from build123d import *

# Parameters (mm, degrees)
CROQUIS2_R            = 1.7
CORTAR_EXTRUIR1_DEPTH = 59
MATRIZC1_COUNT        = 3


with BuildPart() as part:
    # Croquis1 → Revolución1 (revolve)
    with BuildSketch(Plane.XY):
        Polygon((58.282962044, 6), (58.282962044, 0), (75, 0), (75, 27.5), (55, 27.5), (55, 13), (49, 13), (49, 12.5), align=None)
    revolve(axis=Axis((0, 0, 0), (0, 1, 0)))

    # Croquis2 → Cortar-Extruir1 (cut)
    with BuildSketch(Plane(origin=(0, 27.5, 0), x_dir=(1, 0, 0), z_dir=(0, 1, 0))):
        with Locations((-65, 0)):
            Circle(CROQUIS2_R)
    cortar_extruir1 = extrude(amount=-CORTAR_EXTRUIR1_DEPTH, mode=Mode.SUBTRACT)

    # MatrizC1: Cortar-Extruir1 ×3 about axis
    matrizc1_axis = Axis((0, 0, 0), (0, 1, 0))
    for i in range(1, MATRIZC1_COUNT):
        add(cortar_extruir1.rotate(matrizc1_axis, i * 360 / MATRIZC1_COUNT), mode=Mode.SUBTRACT)


solid = part.part
Design review of the part built by this model. Coordinates are the model's own, in mm. A direction names the side the tool comes from. Coordinates: 2 decimals unless noted, no trailing zeros. Loops run counter-clockwise (first coordinate to the right, second up) from the corner with the lowest first, then second, coordinate; pieces in that order, holes last.
Item 1: Clearance check with flat-ended pins moving along their axes: pin 1 (4 mm diameter, centred on x = -18.5, y = 16.5, fed in from +Z); pin 2 (10 mm diameter, centred on y = 20.5, z = 31.5, fed in from -X); pin 3 (5 mm diameter, centred on y = 18, z = -51.5, fed in from -X); pin 4 (2 mm diameter, centred on x = 32.5, z = 56.29, fed in from -Y). State where each tip first meets the part, or that it passes through.
Completed:
pin 1: stops at z = 73.16
pin 2: stops at x = -70.16
pin 3: stops at x = -56.78
pin 4: passes through
Item 2: Add section B-B (y = 4.25). Write out the cut boundary in (x, z), and give its area (3 significant figures).
Completed:
outline: circle Ø150 at (0, 0); hole circle Ø3.4 at (-65, 0); hole circle Ø116.57 at (0, 0); hole circle Ø3.4 at (32.5, -56.29); hole circle Ø3.4 at (32.5, 56.29)
area: 6,970 mm2
Item 3: Add section A-A (x = 0). Write out the cut boundary in (y, z).
Completed:
outline: (0, -75) - (27.5, -75) - (27.5, -55) - (13, -55) - (13, -49) - (12.5, -49) - (6, -58.28) - (0, -58.28) - close; (0, 58.28) - (6, 58.28) - (12.5, 49) - (13, 49) - (13, 55) - (27.5, 55) - (27.5, 75) - (0, 75) - close
Item 4: Wall thickness on L1, parallel to Z at x = 0, y = 12.6; L2, parallel to Z at x = 32.5, y = 11; L3, parallel to X at y = 4.7, z = 0: over which ranges is each line inside the solid? List them lowest first.
Completed:
L1: z = -75 to -49, 49 to 75
L2: z = -67.59 to -57.99, -54.59 to -39.49, 39.49 to 54.59, 57.99 to 67.59
L3: x = -75 to -66.7, -63.3 to -58.28, 58.28 to 75
Item 5: For faces 1 (the flat face through (-49, 13, 4)), 2 (the flat face through (0, 27.5, -56)), 3 (the cylindrical face through (-46.251, 2.958, 35.464)), list the 3-axis set-ups (+Z, -Z, +X, -X, +Y, -Y) from which the entire face can be reached by the end or side of a thin tool; tool diameter is ignored.
Completed:
face 1: +Y
face 2: +Z, -Z, +X, -X, +Y
face 3: -Y
Item 6: Add section C-C (z = 65.5). Write out the cut boundary in (x, y).
Completed:
outline: (-36.53, 0) - (36.53, 0) - (36.53, 27.5) - (-36.53, 27.5) - close
